```python
from build123d import *

# Parameters (mm, degrees)
SKETCH1_W                                        = 130
SKETCH1_H                                        = 110
BOSS_EXTRUDE1_DEPTH                              = 5
SKETCH2_W                                        = 130
SKETCH2_H                                        = 110
BOSS_EXTRUDE2_DEPTH                              = 50
CBORE_FOR_M3_PAN_HEAD_MACHINE_SCREW1_D           = 3.4
CBORE_FOR_M3_PAN_HEAD_MACHINE_SCREW1_DEPTH       = 7
CBORE_FOR_M3_PAN_HEAD_MACHINE_SCREW1_CBORE_D     = 7
CBORE_FOR_M3_PAN_HEAD_MACHINE_SCREW1_CBORE_DEPTH = 2.4
CBORE_FOR_M3_PAN_HEAD_MACHINE_SCREW1_TIP         = 1.021463052
CBORE_FOR_M3_PAN_HEAD_MACHINE_SCREW2_D           = 3.4
CBORE_FOR_M3_PAN_HEAD_MACHINE_SCREW2_DEPTH       = 7
CBORE_FOR_M3_PAN_HEAD_MACHINE_SCREW2_CBORE_D     = 7
CBORE_FOR_M3_PAN_HEAD_MACHINE_SCREW2_CBORE_DEPTH = 2.4
CBORE_FOR_M3_PAN_HEAD_MACHINE_SCREW2_TIP         = 1.021463052
BOSS_EXTRUDE3_REACH                              = 177.926
SKETCH8_W                                        = 5
SKETCH8_H                                        = 20
SKETCH9_W                                        = 5
SKETCH9_H                                        = 20
BOSS_EXTRUDE4_DEPTH                              = 100
CUT_EXTRUDE2_REACH                               = 180.955
SKETCH10_W                                       = 12
SKETCH10_H                                       = 10
CUT_EXTRUDE3_REACH                               = 180.955
SKETCH11_W                                       = 10
SKETCH11_H                                       = 5
FILLET6_R                                        = 5


with BuildPart() as part:
    # Sketch1 → Boss-Extrude1 (new body)
    with BuildSketch(Plane(origin=(0, 0, 0), x_dir=(1, 0, 0), z_dir=(0, 1, 0))):
        with Locations((65, -55)):
            Rectangle(SKETCH1_W, SKETCH1_H)
    extrude(amount=BOSS_EXTRUDE1_DEPTH)

    # Sketch2 → Boss-Extrude2 (add)
    with BuildSketch(Plane(origin=(0, 5, 0), x_dir=(1, 0, 0), z_dir=(0, 1, 0))):
        with Locations((65, -55)):
            Rectangle(SKETCH2_W, SKETCH2_H)
        Polygon((10, -105), (120, -105), (120, -100), (125, -100), (125, -10), (120, -10), (120, -5), (10, -5), (10, -10), (5, -10), (5, -100), (10, -100), align=None, mode=Mode.SUBTRACT)
    extrude(amount=BOSS_EXTRUDE2_DEPTH)

    # CBORE for M3 Pan Head Machine Screw1
    with Locations(Plane(origin=(0, 55, 0), x_dir=(1, 0, 0), z_dir=(0, 1, 0))):
        with Locations((5, -5), (125, -105), (5, -105), (125, -5)):
            CounterBoreHole(CBORE_FOR_M3_PAN_HEAD_MACHINE_SCREW1_D / 2, CBORE_FOR_M3_PAN_HEAD_MACHINE_SCREW1_CBORE_D / 2, CBORE_FOR_M3_PAN_HEAD_MACHINE_SCREW1_CBORE_DEPTH, depth=CBORE_FOR_M3_PAN_HEAD_MACHINE_SCREW1_DEPTH)
            with Locations((0, 0, -(CBORE_FOR_M3_PAN_HEAD_MACHINE_SCREW1_DEPTH + CBORE_FOR_M3_PAN_HEAD_MACHINE_SCREW1_TIP / 2))):  # 118° drill point
                Cone(0, CBORE_FOR_M3_PAN_HEAD_MACHINE_SCREW1_D / 2, CBORE_FOR_M3_PAN_HEAD_MACHINE_SCREW1_TIP, mode=Mode.SUBTRACT)

    # CBORE for M3 Pan Head Machine Screw2
    with Locations(Plane(origin=(0, 0, 0), x_dir=(-1, 0, 0), z_dir=(0, -1, 0))):
        with Locations((-74.07, -75.08), (-72.8, -26.82), (-22.538761246, -62.532927336), (-21.069252595, -34.631598616)):
            CounterBoreHole(CBORE_FOR_M3_PAN_HEAD_MACHINE_SCREW2_D / 2, CBORE_FOR_M3_PAN_HEAD_MACHINE_SCREW2_CBORE_D / 2, CBORE_FOR_M3_PAN_HEAD_MACHINE_SCREW2_CBORE_DEPTH, depth=CBORE_FOR_M3_PAN_HEAD_MACHINE_SCREW2_DEPTH)
            with Locations((0, 0, -(CBORE_FOR_M3_PAN_HEAD_MACHINE_SCREW2_DEPTH + CBORE_FOR_M3_PAN_HEAD_MACHINE_SCREW2_TIP / 2))):  # 118° drill point
                Cone(0, CBORE_FOR_M3_PAN_HEAD_MACHINE_SCREW2_D / 2, CBORE_FOR_M3_PAN_HEAD_MACHINE_SCREW2_TIP, mode=Mode.SUBTRACT)

    # Boss-Extrude3: up to this face of the body (flat: up to its plane)
    boss_extrude3_end = Plane(part.part.faces().sort_by_distance((65, 30, 105))[0])
    # Sketch8 → Boss-Extrude3 (add, up to the picked face)
    with BuildSketch(Plane.XY.offset(5), mode=Mode.PRIVATE) as boss_extrude3_sk1:
        with Locations((117.5, 15)):
            Rectangle(SKETCH8_W, SKETCH8_H)
    boss_extrude3_tool1 = split(extrude(boss_extrude3_sk1.sketch, amount=BOSS_EXTRUDE3_REACH, mode=Mode.PRIVATE), bisect_by=boss_extrude3_end, keep=Keep.BOTH, mode=Mode.PRIVATE)
    add(boss_extrude3_tool1.solids().sort_by(Axis((117.5, 15, 5), (0, 0, 1)))[0])

    # Sketch9 → Boss-Extrude4 (add)
    with BuildSketch(Plane.XY.offset(5)):
        with Locations((12.5, 15)):
            Rectangle(SKETCH9_W, SKETCH9_H)
    extrude(amount=BOSS_EXTRUDE4_DEPTH)

    # Sketch10 → Cut-Extrude2 (cut, up to next)
    with BuildSketch(Plane.XY.offset(110), mode=Mode.PRIVATE) as cut_extrude2_sk1:
        with Locations((104, 15)):
            Rectangle(SKETCH10_W, SKETCH10_H)
    cut_extrude2_tool1 = extrude(cut_extrude2_sk1.sketch, amount=-CUT_EXTRUDE2_REACH, mode=Mode.PRIVATE) & part.part
    add(cut_extrude2_tool1.solids().sort_by_distance((104, 15, 110))[0], mode=Mode.SUBTRACT)

    # Sketch11 → Cut-Extrude3 (cut, up to next)
    with BuildSketch(Plane.XY.offset(110), mode=Mode.PRIVATE) as cut_extrude3_sk1:
        with Locations((105, 37.5)):
            Rectangle(SKETCH11_W, SKETCH11_H)
    cut_extrude3_tool1 = extrude(cut_extrude3_sk1.sketch, amount=-CUT_EXTRUDE3_REACH, mode=Mode.PRIVATE) & part.part
    add(cut_extrude3_tool1.solids().sort_by_distance((105, 37.5, 110))[0], mode=Mode.SUBTRACT)

    # Fillet6
    fillet6_edges = [part.edges().sort_by_distance(p)[0] for p in [
        (0, 27.5, 0),
        (130, 27.5, 0),
        (130, 27.5, 110),
        (0, 27.5, 110),
    ]]
    fillet(fillet6_edges, radius=FILLET6_R)


solid = part.part
```
The listing builds one solid part. Answer for the finished solid, in the listing's coordinates (mm). A direction names the side the tool comes from. Give positions to 0.01 mm unless a question says otherwise; leave off trailing zeros. Order: outer loops, then holes, each group sorted by start corner. A loop starts at its lowest first (then second) coordinate and runs counter-clockwise, first axis right, second up.
1) Find section A-A on z = 75.08. Write down the section's boundary in (x, y), then the cut area to 3 significant figures.
Reported:
outline: (0, 0) - (70.57, 0) - (70.57, 2.4) - (72.37, 2.4) - (72.37, 5) - (15, 5) - (15, 25) - (10, 25) - (10, 5) - (5, 5) - (5, 55) - (0, 55) - close; (75.77, 2.4) - (77.57, 2.4) - (77.57, 0) - (130, 0) - (130, 55) - (125, 55) - (125, 5) - (120, 5) - (120, 25) - (115, 25) - (115, 5) - (75.77, 5) - close
area: 1,320 mm2
2) Find section C-C on y = 13. Write down the section's boundary in (x, z), then the cut area to 3 significant figures.
Reported:
outline: (0, 5) arc R5 ccw to (5, 0) - (125, 0) arc R5 ccw to (130, 5) - (130, 105) arc R5 ccw to (125, 110) - (110, 110) - (110, 105) - (115, 105) - (115, 5) - (15, 5) - (15, 105) - (98, 105) - (98, 110) - (5, 110) arc R5 ccw to (0, 105) - close; hole (5, 10) - (10, 10) - (10, 100) - (5, 100) - close; hole (120, 10) - (125, 10) - (125, 100) - (120, 100) - close
area: 3,320 mm2
3) Determine the mould class of faces 1 (the face through (1, 28, 108)), 2 (the face through (130, 27, 56)), 3 (the face through (65, 55, 2)), 4 (the face through (20, 2.4, 33)) for opening direction X: pulls with the +X half, pulls with the -X half, needs draft (parallel to the pull), parting line crosses it, or undercut.
Reported:
face 1: pulls with the -X half
face 2: pulls with the +X half
face 3: needs draft
face 4: undercut
4) Find section B-B on y = 44. Write down the section's boundary in (x, z).
Reported:
outline: (0, 5) arc R5 ccw to (5, 0) - (125, 0) arc R5 ccw to (130, 5) - (130, 105) arc R5 ccw to (125, 110) - (5, 110) arc R5 ccw to (0, 105) - close; hole (5, 10) - (10, 10) - (10, 5) - (120, 5) - (120, 10) - (125, 10) - (125, 100) - (120, 100) - (120, 105) - (10, 105) - (10, 100) - (5, 100) - close
5) Given P1, Ø3.5, axis at x = 124.5, z = 6, coming from the +Y side; P2, Ø4, axis at y = 12.5, z = 108, coming from the -X side; P3, Ø3, axis at x = 37, z = 44.5, coming from the -Y side; P4, Ø2.5, axis at x = 22.54, z = 62.53, coming from the -Y side, each flat-ended and moving along its own axis, determine where each tip first touches the part or whether it passes through.
Reported:
P1: stops at y = 52.6
P2: stops at x = 0.1
P3: stops at y = 0
P4: passes through
6) For faces 5 (the face through (19.454, 1.183, 37.737)), 6 (the face through (64, 27, 110)), 7 (the face through (66, 30, 5)), determine the directions among +Z, -Z, +X, -X, +Y, -Y from which every point of the face is accessible in a straight line to the end or side of a thin tool.
Reported:
face 5: -Y
face 6: +Z, +X, -X, +Y, -Y
face 7: +Y
7) Consider line 1 along X through (y, z) = (13, 77); line 2 along X through (y, z) = (49, 61); line 3 along Z through (x, y) = (105.5, 22.5). Determine where each line is inside the solid, lowest interval first.
Reported:
line 1: x = 0 to 5, 10 to 15, 115 to 120, 125 to 130
line 2: x = 0 to 5, 125 to 130
line 3: z = 0 to 5, 105 to 110
8) Find section D-D on z = 45. Write down the section's boundary in (x, y).
Reported:
outline: (0, 0) - (130, 0) - (130, 55) - (125, 55) - (125, 5) - (120, 5) - (120, 25) - (115, 25) - (115, 5) - (15, 5) - (15, 25) - (10, 25) - (10, 5) - (5, 5) - (5, 55) - (0, 55) - close
